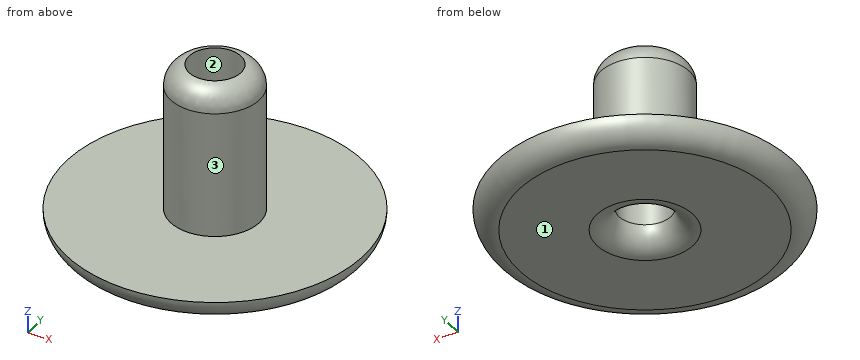
```python
from build123d import *

# Parameters (mm, degrees)
F0_R     = 10
F1_DEPTH = 1.5
F2_R     = 3
F3_DEPTH = 10
F4_R     = 1.75
F5_DEPTH = 11.501


# Not quite as in the source:
# - a fillet or chamfer that OpenCascade refuses, or shapes differently, is made with other operations: its cross-section is extruded or revolved along the edge and cut away or added


with BuildPart() as f1:
    # F0 (on Top) → F1 (new body)
    with BuildSketch(Plane.XY):
        Circle(F0_R)
    extrude(amount=F1_DEPTH)

    # F2 (on face) → F3 (join)
    with BuildSketch(Plane.XY.offset(1.5)):
        Circle(F2_R)
    extrude(amount=F3_DEPTH)

    # F4 (on face) → F5 (cut, through all)
    with BuildSketch(Plane.XY.offset(11.5)):
        Circle(F4_R)
    extrude(amount=-F5_DEPTH, mode=Mode.SUBTRACT)

    # F6: fillet of radius 1.5 on 3 edges, made by hand

    # F6_s1 → F6_t2 (revolve, cut)
    with BuildSketch(Plane.XZ):
        with BuildLine():
            ThreePointArc((10, 1.5), (9.5606601718, 0.4393398282), (8.5, 0))
            Line((8.5, 0), (10, 0))
            Line((10, 0), (10, 1.5))
        make_face()
    revolve(axis=Axis((0, 0, 0), (0, 0, 1)), mode=Mode.SUBTRACT)

    # F6_s3 → F6_t4 (revolve, cut)
    with BuildSketch(Plane.XZ):
        with BuildLine():
            ThreePointArc((3.25, 0), (2.1893398282, 0.4393398282), (1.75, 1.5))
            Line((1.75, 1.5), (1.75, 0))
            Line((1.75, 0), (3.25, 0))
        make_face()
    revolve(axis=Axis((0, 0, 0), (0, 0, 1)), mode=Mode.SUBTRACT)

    # F6_s5 → F6_t6 (revolve, cut)
    with BuildSketch(Plane.XZ):
        with BuildLine():
            ThreePointArc((3, 10.0209800542), (2.6456439237, 10.9892258908), (1.75, 11.5))
            Line((1.75, 11.5), (3, 11.5))
            Line((3, 11.5), (3, 10.0209800542))
        make_face()
    revolve(axis=Axis((0, 0, 11.5), (0, 0, 1)), mode=Mode.SUBTRACT)


solid = f1.part
```
CAD build for the part. Positions are in the model's coordinates, mm. Face numbers are marked on the shaded views. Coordinates: 2 decimals unless noted, no trailing zeros. Write each loop counter-clockwise with the first axis right and the second up, starting at its lowest first coordinate (ties: lowest second). Pieces come first, ordered by that corner, then holes. Notation, with made-up numbers: (51, 25.5) -> (78, 25.5) arc R21 cw to (78, 63.5) -> close; hole circle Ø10 at (63.5, -0.75). An arc over 180 degrees is marked (long way). Return JSON: item names as keys, results as strings. Group by question number.
Q1. Cut at A-A, the plane z = 4. Give the cut face in (x, y).
Q2. Pull direction X, two halves, no side cores. Call the marked faces 1, 2 and 3: released by +X, released by -X, zero draft, split by the parting line, or undercut.
Q3. Flat gauge pins, fed straight in: pin 1 (3 mm diameter, centred on x = 0, y = 0, fed in from -Z); pin 2 (1.5 mm diameter, centred on y = -1.5, z = 8.5, fed in from -X). Where does each tip first touch, or does it go through?
Q4. Drill centre lines: line 1 (Y direction, x = 0, z = 3.5); line 2 (Z direction, x = -0.5, y = 6.25); line 3 (X direction, y = 1, z = 9.5). Where is each one in solid material? Low to high.
Returned:
{
 "1": {"outline": "circle Ø6 at (0, 0); hole circle Ø3.5 at (0, 0)"},
 "2": {"face 1": "zero draft", "face 2": "undercut", "face 3": "split by the parting line"},
 "3": {"pin 1": "passes through", "pin 2": "stops at x = -2.9"},
 "4": {"line 1": "y = -3 to -1.75, 1.75 to 3", "line 2": "z = 0 to 1.5", "line 3": "x = -2.83 to -1.44, 1.44 to 2.83"}
}
